Geometry: see drawing. Coordinates: mm, zero at the bounding-box minimum. Round coordinates to 2 decimals unless told otherwise and drop trailing zeros. Loops run counter-clockwise (first coordinate to the right, second up) from the corner with the lowest first, then second, coordinate; pieces in that order, holes last. Notation, with made-up numbers: (-17, 14) - (-12, 14) arc R17 cw to (-12, 41) - close; hole circle Ø9 at (38, -31). An arc over 180 degrees is marked (long way). Answer in a Markdown table with one row per item. Add a question column.
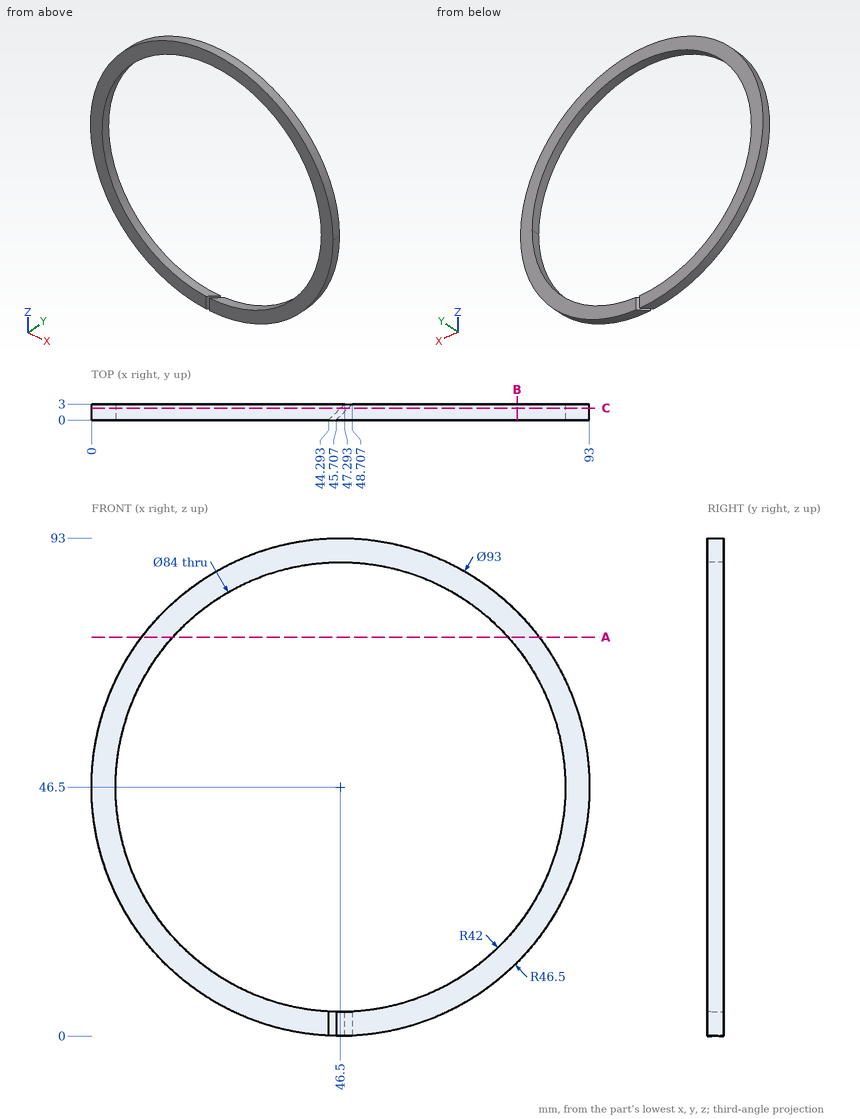
1) Section B-B, the plane x = 79.5. Return the cut outline in (y, z), and give its area (3 significant figures).
2) Section A-A, the plane z = 74.5. Return the cut outline in (x, y) (3 decimals), and give its area (3 significant figures).
3) Section C-C, the plane y = 2.25. Return the cut outline in (x, z), and give its area (3 significant figures).
4) Contact query for flat-ended pins moving along their axis: pin 1 Ø1 at (y, z) = (2.5, 74.5) entering from -X; pin 2 Ø1 at (y, z) = (2, 79) entering from +X; pin 3 Ø1.5 at (x, y) = (71, 2.5) entering from -Z. Output: stop coordinate, or through.
5) Material intervals for line 1 along X through (y, z) = (1.9, 46.5); line 2 along X through (y, z) = (1.9, 82) (1 decimal), sorted ascending. Write a range as from..to.
Evaluation:
| question | item | result |
|---|---|---|
| 1 | outline | (0, 13.74) - (3, 13.74) - (3, 20.52) - (0, 20.52) - close; (0, 72.48) - (3, 72.48) - (3, 79.26) - (0, 79.26) - close |
| 1 | area | 40.7 mm² |
| 2 | outline | (9.375, 0) - (15.195, 0) - (15.195, 3) - (9.375, 3) - close; (77.805, 0) - (83.625, 0) - (83.625, 3) - (77.805, 3) - close |
| 2 | area | 34.9 mm² |
| 3 | outline | (46.54, 0) - (46.54, 4.5) arc R42 cw (long way) to (47.96, 4.53) - (47.96, 0.02) arc R46.5 ccw (long way) to start |
| 3 | area | 1,240 mm² |
| 4 | pin 1 | stops at x = 9 |
| 4 | pin 2 | stops at x = 80.24 |
| 4 | pin 3 | stops at z = 6.52 |
| 5 | line 1 | x = 0..4.5, 88.5..93 |
| 5 | line 2 | x = 16.5..24.1, 68.9..76.5 |
